from build123d import *

# Parameters (mm, degrees)
F0_W      = 55
F0_H      = 58
F1_DEPTH  = 4
F2_W      = 55
F2_H      = 58
F2_W_2    = 47
F2_H_2    = 50
F3_DEPTH  = 8
F4_R      = 2
F5_W      = 10
F5_H      = 10
F6_DEPTH  = 25.4
F7_W      = 10
F7_H      = 4
F8_DEPTH  = 17.018
F9_R      = 1
F11_DEPTH = 4
F13_DEPTH = 12
F14_R     = 2.5
F15_DEPTH = 4
F16_R     = 1.5
F17_DEPTH = 25.4


# Not quite as in the source:
# - a feature names something its author has since deleted; it is built from what else it names


with BuildPart() as f1:
    # F0 (on Top) → F1 (new body)
    with BuildSketch(Plane.XY):
        Rectangle(F0_W, F0_H)
    extrude(amount=F1_DEPTH)

    # F2 (on face) → F3 (join)
    with BuildSketch(Plane.XY.offset(4)):
        Rectangle(F2_W, F2_H)
        Rectangle(F2_W_2, F2_H_2, mode=Mode.SUBTRACT)
    extrude(amount=F3_DEPTH)

    # F4
    f4_edges = [f1.edges().sort_by_distance(p)[0] for p in [
        (23.5, -25, 8),
        (-23.5, -25, 8),
        (-23.5, 25, 8),
        (23.5, 25, 8),
    ]]
    fillet(f4_edges, radius=F4_R)

    # F5 (on face) → F6 (cut)
    with BuildSketch(Plane.XY.offset(12)):
        with Locations((-16.5, -20)):
            Rectangle(F5_W, F5_H)
    extrude(amount=-F6_DEPTH, mode=Mode.SUBTRACT)

    # F7 (on face) → F8 (cut)
    with BuildSketch(Plane.XY.offset(12)):
        with Locations((-16.5, -27)):
            Rectangle(F7_W, F7_H)
    extrude(amount=-F8_DEPTH, mode=Mode.SUBTRACT)

    # F9
    f9_edges = [f1.edges().sort_by_distance(p)[0] for p in [
        (-21.5, -15, 2),
        (-11.5, -15, 2),
    ]]
    fillet(f9_edges, radius=F9_R)

    # F10 (on face) → F11 (cut)
    with BuildSketch(Plane.XY.offset(12)):
        with BuildLine():
            Line((25.5, -27), (25.5, 27))
            Line((25.5, 27), (-25.5, 27))
            Line((-25.5, 27), (-25.5, -27))
            Line((-25.5, -27), (-21.5, -27))
            Line((-21.5, -27), (-21.5, -25))
            ThreePointArc((-21.5, -25), (-22.9142135624, -24.4142135624), (-23.5, -23))
            Line((-23.5, -23), (-23.5, 23))
            ThreePointArc((-23.5, 23), (-22.9142135624, 24.4142135624), (-21.5, 25))
            Line((-21.5, 25), (21.5, 25))
            ThreePointArc((21.5, 25), (22.9142135624, 24.4142135624), (23.5, 23))
            Line((23.5, 23), (23.5, -23))
            ThreePointArc((23.5, -23), (22.9142135624, -24.4142135624), (21.5, -25))
            Line((21.5, -25), (-11.5, -25))
            Line((-11.5, -25), (-11.5, -27))
            Line((-11.5, -27), (25.5, -27))
        make_face()
    extrude(amount=-F11_DEPTH, mode=Mode.SUBTRACT)

    # F12 (on face) → F13 (join)
    with BuildSketch(Plane(origin=(0, 0, 0), x_dir=(1, 0, 0), z_dir=(0, 0, -1))):
        with BuildLine():
            ThreePointArc((-26.0358983849, 29), (-25.6362966948, 29.9647238196), (-25.5, 31))
            ThreePointArc((-25.5, 31), (-25.7257453718, 32.3247648854), (-26.3775010008, 33.5))
            Line((-26.3775010008, 33.5), (-32, 33.5))
            Line((-32, 33.5), (-32, 27.8775010008))
            ThreePointArc((-32, 27.8775010008), (-29.8027756377, 27.011475597), (-27.5, 27.5358983849))
            Line((-27.5, 27.5358983849), (-27.5, 29))
            Line((-27.5, 29), (-26.0358983849, 29))
        make_face()
        with BuildLine():
            Line((-32, 33.5), (-26.3775010008, 33.5))
            ThreePointArc((-26.3775010008, 33.5), (-32.3284271247, 33.8284271247), (-32, 27.8775010008))
            Line((-32, 27.8775010008), (-32, 33.5))
        make_face()
        with BuildLine():
            ThreePointArc((-27.5, 27.5358983849), (-29.8027756377, 27.011475597), (-32, 27.8775010008))
            Line((-32, 27.8775010008), (-27.5, 23.1462475253))
            Line((-27.5, 23.1462475253), (-27.5, 27.5358983849))
        make_face()
        with BuildLine():
            ThreePointArc((-26.3775010008, 33.5), (-25.7257453718, 32.3247648854), (-25.5, 31))
            ThreePointArc((-25.5, 31), (-25.6362966948, 29.9647238196), (-26.0358983849, 29))
            Line((-26.0358983849, 29), (-22.0974513047, 29))
            Line((-22.0974513047, 29), (-26.3775010008, 33.5))
        make_face()
        with BuildLine():
            Line((32, 33.5), (26.3775010008, 33.5))
            ThreePointArc((26.3775010008, 33.5), (25.511475597, 31.3027756377), (26.0358983849, 29))
            Line((26.0358983849, 29), (27.5, 29))
            Line((27.5, 29), (27.5, 27.5358983849))
            ThreePointArc((27.5, 27.5358983849), (29.8027756377, 27.011475597), (32, 27.8775010008))
            Line((32, 27.8775010008), (32, 33.5))
        make_face()
        with BuildLine():
            ThreePointArc((33.5, 31), (30.8247648854, 34.7742546282), (26.3775010008, 33.5))
            Line((26.3775010008, 33.5), (32, 33.5))
            Line((32, 33.5), (32, 27.8775010008))
            ThreePointArc((32, 27.8775010008), (33.1055512755, 29.2679491924), (33.5, 31))
        make_face()
        with BuildLine():
            Line((27.5, 23.1462475253), (32, 27.8775010008))
            ThreePointArc((32, 27.8775010008), (29.8027756377, 27.011475597), (27.5, 27.5358983849))
            Line((27.5, 27.5358983849), (27.5, 23.1462475253))
        make_face()
        with BuildLine():
            ThreePointArc((26.0358983849, 29), (25.511475597, 31.3027756377), (26.3775010008, 33.5))
            Line((26.3775010008, 33.5), (22.0974513047, 29))
            Line((22.0974513047, 29), (26.0358983849, 29))
        make_face()
        with BuildLine():
            ThreePointArc((-27.5, -27.5358983849), (-29.8027756377, -27.011475597), (-32, -27.8775010008))
            Line((-32, -27.8775010008), (-32, -33.5))
            Line((-32, -33.5), (-26.3775010008, -33.5))
            ThreePointArc((-26.3775010008, -33.5), (-25.7257453718, -32.3247648854), (-25.5, -31))
            ThreePointArc((-25.5, -31), (-25.6362966948, -29.9647238196), (-26.0358983849, -29))
            Line((-26.0358983849, -29), (-27.5, -29))
            Line((-27.5, -29), (-27.5, -27.5358983849))
        make_face()
        with BuildLine():
            Line((-32, -33.5), (-32, -27.8775010008))
            ThreePointArc((-32, -27.8775010008), (-32.3284271247, -33.8284271247), (-26.3775010008, -33.5))
            Line((-26.3775010008, -33.5), (-32, -33.5))
        make_face()
        with BuildLine():
            Line((-27.5, -23.1462475253), (-32, -27.8775010008))
            ThreePointArc((-32, -27.8775010008), (-29.8027756377, -27.011475597), (-27.5, -27.5358983849))
            Line((-27.5, -27.5358983849), (-27.5, -23.1462475253))
        make_face()
        with BuildLine():
            ThreePointArc((-25.5, -31), (-25.7257453718, -32.3247648854), (-26.3775010008, -33.5))
            Line((-26.3775010008, -33.5), (-22.0974513047, -29))
            Line((-22.0974513047, -29), (-26.0358983849, -29))
            ThreePointArc((-26.0358983849, -29), (-25.6362966948, -29.9647238196), (-25.5, -31))
        make_face()
        with BuildLine():
            ThreePointArc((26.0358983849, -29), (25.511475597, -31.3027756377), (26.3775010008, -33.5))
            Line((26.3775010008, -33.5), (32, -33.5))
            Line((32, -33.5), (32, -27.8775010008))
            ThreePointArc((32, -27.8775010008), (29.8027756377, -27.011475597), (27.5, -27.5358983849))
            Line((27.5, -27.5358983849), (27.5, -29))
            Line((27.5, -29), (26.0358983849, -29))
        make_face()
        with BuildLine():
            Line((22.0974513047, -29), (26.3775010008, -33.5))
            ThreePointArc((26.3775010008, -33.5), (25.511475597, -31.3027756377), (26.0358983849, -29))
            Line((26.0358983849, -29), (22.0974513047, -29))
        make_face()
        with BuildLine():
            ThreePointArc((27.5, -27.5358983849), (29.8027756377, -27.011475597), (32, -27.8775010008))
            Line((32, -27.8775010008), (27.5, -23.1462475253))
            Line((27.5, -23.1462475253), (27.5, -27.5358983849))
        make_face()
        with BuildLine():
            Line((32, -33.5), (26.3775010008, -33.5))
            ThreePointArc((26.3775010008, -33.5), (30.8247648854, -34.7742546282), (33.5, -31))
            ThreePointArc((33.5, -31), (33.1055512755, -29.2679491924), (32, -27.8775010008))
            Line((32, -27.8775010008), (32, -33.5))
        make_face()
    extrude(amount=-F13_DEPTH)

    # F14 (on face) → F15 (cut)
    with BuildSketch(Plane(origin=(0, 0, 0), x_dir=(1, 0, 0), z_dir=(0, 0, -1))):
        with Locations((-29.5, -31)):
            Circle(F14_R)
        with Locations((29.5, -31)):
            Circle(F14_R)
        with Locations((-29.5, 31)):
            Circle(F14_R)
        with Locations((29.5, 31)):
            Circle(F14_R)
    extrude(amount=-F15_DEPTH, mode=Mode.SUBTRACT)

    # F16 (on face) → F17 (cut)
    with BuildSketch(Plane.XY.offset(12)):
        with Locations((29.5, -31)):
            Circle(F16_R)
        with Locations((-29.5, -31)):
            Circle(F16_R)
        with Locations((29.5, 31)):
            Circle(F16_R)
        with Locations((-29.5, 31)):
            Circle(F16_R)
    extrude(amount=-F17_DEPTH, mode=Mode.SUBTRACT)


solid = f1.part
The listing builds one solid part. Answer for the finished solid, in the listing's coordinates (mm). A direction names the side the tool comes from. Round coordinates to 2 decimals unless told otherwise and drop trailing zeros. Write each loop counter-clockwise with the first axis right and the second up, starting at its lowest first coordinate (ties: lowest second). Pieces come first, ordered by that corner, then holes. Notation, with made-up numbers: (29, -36) - (77, -36) arc R17 cw to (77, -30) - close; hole circle Ø1 at (30.5, 84). An arc over 180 degrees is marked (long way). Use a Markdown table: item, result. Add a question column.
1. A tool of negligible diameter and unlimited length cuts with its end or side. For faces 5 (the face through (24, -31, 6)), 6 (the face through (-27.5, 0, 6)), 7 (the face through (22.93, -24.4, 6.03)), 8 (the face through (29.17, 28.52, 1.97)), from which of +Z, -Z, +X, -X, +Y, -Y can it reach the whole face along a straight path? Write none if from no direction.
2. Consider line 1 (Y direction, x = -29.5, z = 1.55); line 2 (X direction, y = 19, z = 7); line 3 (X direction, y = -31, z = 2.65). Determine where each line is inside the solid, lowest interval first.
3. The part is cut by section D-D (x = -29). Write down the section's boundary in (y, z).
4. The part is cut by section C-C (z = 5.25). Give the number of separate pieces and of enclosed holes in the cut face, and give its area (3 significant figures).
5. The part is cut by section B-B (x = 4). Write down the section's boundary in (y, z).
6. The part is cut by section A-A (y = -17). Write down the section's boundary in (x, z), and give its area (3 significant figures).
7. Flat-ended cylindrical pins translate along their axes: P1, Ø3, axis at y = -22.5, z = 10.5, coming from the +X side; P2, Ø1.5, axis at y = -8.5, z = 10, coming from the +X side; P3, Ø1.5, axis at x = 22.5, z = 5.5, coming from the +Y side. Find the tip coordinate at first contact, or state that the pin passes through.
8. For a pull along Y with two mould halves and no side action, classify faces 1 (the face through (-24, -31, 6)), 2 (the face through (2, 28, 12)), 3 (the face through (0, 29, 6)), 4 (the face through (-29.83, 28.52, 1.97)) as +Y half, -Y half, draft (parallel to the pull), parting line (faces both ways), or undercut.
Reported:
| question | item | result |
|---|---|---|
| 1 | face 5 | +Z, -Z, -Y |
| 1 | face 6 | +Z, -Z, -X |
| 1 | face 7 | +Z |
| 1 | face 8 | -Z |
| 2 | line 1 | -35 to -33.5, -28.5 to -25.25, 25.25 to 28.5, 33.5 to 35 |
| 2 | line 2 | -27.5 to -23.5, 23.5 to 27.5 |
| 2 | line 3 | -33.5 to -32, -27 to -24, 24 to 27, 32 to 33.5 |
| 3 | outline | (-34.97, 0) - (-33.45, 0) - (-33.45, 4) - (-32.41, 4) - (-32.41, 12) - (-34.97, 12) - close; (-29.59, 4) - (-28.55, 4) - (-28.55, 0) - (-24.72, 0) - (-24.72, 12) - (-29.59, 12) - close; (24.72, 0) - (28.55, 0) - (28.55, 4) - (29.59, 4) - (29.59, 12) - (24.72, 12) - close; (32.41, 4) - (33.45, 4) - (33.45, 0) - (34.97, 0) - (34.97, 12) - (32.41, 12) - close |
| 4 | separate pieces | 1 |
| 4 | enclosed holes | 4 |
| 4 | area | 1,030 mm^2 |
| 5 | outline | (-29, 0) - (29, 0) - (29, 12) - (27, 12) - (27, 8) - (25, 8) - (25, 4) - (-25, 4) - (-25, 8) - (-27, 8) - (-27, 12) - (-29, 12) - close |
| 6 | outline | (-27.5, 0) - (-21.5, 0) - (-21.5, 4) - (-23.5, 4) - (-23.5, 8) - (-25.5, 8) - (-25.5, 12) - (-27.5, 12) - close; (-11.5, 0) - (27.5, 0) - (27.5, 12) - (25.5, 12) - (25.5, 8) - (23.5, 8) - (23.5, 4) - (-11.5, 4) - close |
| 6 | area | 228 mm^2 |
| 7 | P1 | x = 28.31 |
| 7 | P2 | x = 27.5 |
| 7 | P3 | y = 30.21 |
| 8 | face 1 | -Y half |
| 8 | face 2 | draft |
| 8 | face 3 | +Y half |
| 8 | face 4 | undercut |
